Verification items for the finished model (mm, model axes). A direction names the side the tool comes from. Coordinates: 2 decimals unless noted, no trailing zeros. Answer as a JSON object with one key per item and string values. Group by question number.
(1) Material ranges on line 1 (X direction, y = -17, z = -2); line 2 (Y direction, x = -9, z = -3); line 3 (X direction, y = 10, z = -2.5), recorded low to high.
(2) Cross-section at A-A (z = -1.5). Count the separate pieces of the cut face and the enclosed holes in it, plus the area to 3 significant figures.
(3) Mould release check, pull along X, two halves, no side actions. Record for faces 4 (the face through (-14, 18, 0)), 5 (the face through (16.467, -18.072, 0.056)), 6 (the face through (21.68, 3.13, -3.57)): released by +X, released by -X, zero draft, split by the parting line, or undercut.
(4) Access from +Z, -Z, +X, -X, +Y, -Y to the whole of each face (thin tool, end or side, straight path). Record for faces 1 (the face through (-8.53, -21.09, 0.04)), 2 (the face through (4.972, -13.295, 0.056)), 3 (the face through (8.381, -20.484, -3.572)).
(5) Gauge pin test, flat ends, axial feed: pin 1 Ø2 at (x, z) = (-28, -1.5) entering from +Y; pin 2 Ø2.5 at (y, z) = (2, 0) entering from +X; pin 3 Ø4 at (x, z) = (26, -0.5) entering from +Y; pin 4 Ø20 at (x, y) = (0, 0) entering from +Z. Record the tip position at first contact, or that the pin passes through.
from build123d import *

# Parameters (mm, degrees)
F0_R     = 11.05
F1_DEPTH = 4
F2_COUNT = 3
F3_R     = 1.5


with BuildPart() as f1:
    # F0 (on Top) → F1 (new body, symmetric)
    with BuildSketch(Plane.XY):
        with BuildLine():
            Line((-14, 27.5), (-14, 0))
            ThreePointArc((-14, 0), (0, -14), (14, 0))
            Line((14, 0), (14, 27.5))
            ThreePointArc((14, 27.5), (0, 41.5), (-14, 27.5))
        make_face()
        Circle(F0_R, mode=Mode.SUBTRACT)
        with BuildLine():
            Line((-11.05, 8.5963655111), (-11.05, 18.9036344889))
            ThreePointArc((-11.05, 18.9036344889), (-7.3111120124, 15.5606683126), (-2.6339134382, 13.75))
            ThreePointArc((-2.6339134382, 13.75), (-7.3111120124, 11.9393316874), (-11.05, 8.5963655111))
        make_face(mode=Mode.SUBTRACT)
        Polygon((-9.8438220897, 27.5), (-4.9219110448, 36.025), (4.9219110448, 36.025), (9.8438220897, 27.5), (4.9219110448, 18.975), (-4.9219110448, 18.975), align=None, mode=Mode.SUBTRACT)
        with BuildLine():
            Line((11, 18.8397459622), (11, 8.6602540378))
            ThreePointArc((11, 8.6602540378), (7.2764879853, 11.9604649826), (2.6339134382, 13.75))
            ThreePointArc((2.6339134382, 13.75), (7.2764879853, 15.5395350174), (11, 18.8397459622))
        make_face(mode=Mode.SUBTRACT)
    extrude(amount=F1_DEPTH, both=True)

    # F2: F1 ×3 about axis
    f2_axis = Axis((0, 0, 4), (0, 0, 1))


with BuildPart() as f1_1:
    add(f1.part)
    for i in range(1, F2_COUNT):
        add(f1.part.rotate(f2_axis, i * 360 / F2_COUNT))

    # F3
    f3_edges = [f1_1.edges().sort_by_distance(p)[0] for p in [
        (14, 27.5, 0),
        (0, 41.5, -4),
        (-14, 27.5, 0),
        (0, 41.5, 4),
        (16.815699, -25.874356, 0),
        (35.940054, -20.75, -4),
        (30.815699, -1.625644, 0),
        (35.940054, -20.75, 4),
        (-30.815699, -1.625644, 0),
        (-35.940054, -20.75, -4),
        (-16.815699, -25.874356, 0),
        (-35.940054, -20.75, 4),
    ]]
    fillet(f3_edges, radius=F3_R)


solid = f1_1.part
Taken from the geometry:
{
 "1": {"line 1": "x = -37.43 to -31.78, -15.85 to -10.2, -7.34 to -1.44, 1.44 to 7.44, 10.2 to 15.85, 31.78 to 37.43", "line 2": "y = -21.26 to -17.96, -10.72 to -6.41, 6.41 to 10.97, 16.78 to 26.04, 28.96 to 38.11", "line 3": "x = -14 to -11.05, -10.68 to -4.7, 4.7 to 10.68, 11 to 14"},
 "2": {"separate pieces": "1", "enclosed holes": "10", "area": "1,580 mm²"},
 "3": {"face 4": "released by -X", "face 5": "undercut", "face 6": "released by +X"},
 "4": {"face 1": "+Z, -Z, -Y", "face 2": "+Z, -Z", "face 3": "-Z, -Y"},
 "5": {"pin 1": "stops at y = 0.58", "pin 2": "stops at x = 26.7", "pin 3": "stops at y = 2.31", "pin 4": "passes through"}
}
